```python
from build123d import *

# Parameters (mm, degrees)
CUT_EXTRUDE1_REACH = 60.936
SKETCH2_R          = 2.5


with BuildPart() as part:
    # Sketch1 → Revolve1 (revolve)
    with BuildSketch(Plane(origin=(0, 0, 0), x_dir=(1, 0, 0), z_dir=(0, 1, 0)), mode=Mode.PRIVATE) as revolve1_sk:
        Polygon((0, 0), (0, 28.5), (4, 28.5), (4, 14), (19, 14), (19, 6), (43, 6), (43, 0), align=None)
    revolve(revolve1_sk.sketch.rotate(Axis((-51.704391892, 0, 0), (1, 0, 0)), 180), axis=Axis((-51.704391892, 0, 0), (1, 0, 0)))

    # Sketch2 → Cut-Extrude1 (cut, up to next)
    with BuildSketch(Plane.ZY, mode=Mode.PRIVATE) as cut_extrude1_sk1:
        with Locations((0, 23.75)):
            Circle(SKETCH2_R)
    cut_extrude1_tool1 = extrude(cut_extrude1_sk1.sketch, amount=-CUT_EXTRUDE1_REACH, mode=Mode.PRIVATE) & part.part
    # Sketch2 → Cut-Extrude1 (cut, up to next)
    with BuildSketch(Plane.ZY, mode=Mode.PRIVATE) as cut_extrude1_sk2:
        with Locations((20.56810334, 11.875)):
            Circle(SKETCH2_R)
    cut_extrude1_tool2 = extrude(cut_extrude1_sk2.sketch, amount=-CUT_EXTRUDE1_REACH, mode=Mode.PRIVATE) & part.part
    # Sketch2 → Cut-Extrude1 (cut, up to next)
    with BuildSketch(Plane.ZY, mode=Mode.PRIVATE) as cut_extrude1_sk3:
        with Locations((20.56810334, -11.875)):
            Circle(SKETCH2_R)
    cut_extrude1_tool3 = extrude(cut_extrude1_sk3.sketch, amount=-CUT_EXTRUDE1_REACH, mode=Mode.PRIVATE) & part.part
    # Sketch2 → Cut-Extrude1 (cut, up to next)
    with BuildSketch(Plane.ZY, mode=Mode.PRIVATE) as cut_extrude1_sk4:
        with Locations((0, -23.75)):
            Circle(SKETCH2_R)
    cut_extrude1_tool4 = extrude(cut_extrude1_sk4.sketch, amount=-CUT_EXTRUDE1_REACH, mode=Mode.PRIVATE) & part.part
    # Sketch2 → Cut-Extrude1 (cut, up to next)
    with BuildSketch(Plane.ZY, mode=Mode.PRIVATE) as cut_extrude1_sk5:
        with Locations((-20.56810334, -11.875)):
            Circle(SKETCH2_R)
    cut_extrude1_tool5 = extrude(cut_extrude1_sk5.sketch, amount=-CUT_EXTRUDE1_REACH, mode=Mode.PRIVATE) & part.part
    # Sketch2 → Cut-Extrude1 (cut, up to next)
    with BuildSketch(Plane.ZY, mode=Mode.PRIVATE) as cut_extrude1_sk6:
        with Locations((-20.56810334, 11.875)):
            Circle(SKETCH2_R)
    cut_extrude1_tool6 = extrude(cut_extrude1_sk6.sketch, amount=-CUT_EXTRUDE1_REACH, mode=Mode.PRIVATE) & part.part
    add(cut_extrude1_tool1.solids().sort_by_distance((0, 23.75, 0))[0], mode=Mode.SUBTRACT)
    add(cut_extrude1_tool2.solids().sort_by_distance((0, 11.875, 20.568103))[0], mode=Mode.SUBTRACT)
    add(cut_extrude1_tool3.solids().sort_by_distance((0, -11.875, 20.568103))[0], mode=Mode.SUBTRACT)
    add(cut_extrude1_tool4.solids().sort_by_distance((0, -23.75, 0))[0], mode=Mode.SUBTRACT)
    add(cut_extrude1_tool5.solids().sort_by_distance((0, -11.875, -20.568103))[0], mode=Mode.SUBTRACT)
    add(cut_extrude1_tool6.solids().sort_by_distance((0, 11.875, -20.568103))[0], mode=Mode.SUBTRACT)


solid = part.part
```
Input: part model. Units: mm. Frame: model coordinates. A direction names the side the tool comes from. Give positions to 0.01 mm unless a question says otherwise; leave off trailing zeros. Loops run counter-clockwise (first coordinate to the right, second up) from the corner with the lowest first, then second, coordinate; pieces in that order, holes last.
1) Section query C-C on y = 23.75. Return the cut outline in (x, z).
A:
outline: (0, -15.75) - (4, -15.75) - (4, -2.5) - (0, -2.5) - close; (0, 2.5) - (4, 2.5) - (4, 15.75) - (0, 15.75) - close
2) Line query: L1, parallel to X at y = -15, z = 14.5; L2, parallel to X at y = 2, z = 9; L3, parallel to Z at x = 28, y = 4. Output: solid intervals per line, ascending.
A:
L1: x = 0 to 4
L2: x = 0 to 19
L3: z = -4.47 to 4.47
3) Mould query, pull axis Z, two halves, no side actions, for faces 1 (the flat face through (0, 0, 0)), 2 (the cylindrical face through (1.972, 9.657, 21.722)), 3 (the cylindrical face through (11.605, 5.362, 12.932)). Classes: released by +Z, released by -Z, zero draft, split by the parting line, or undercut.
A:
face 1: zero draft
face 2: undercut
face 3: split by the parting line
4) Section query B-B on y = 0. Return the cut outline in (x, z).
A:
outline: (0, -28.5) - (4, -28.5) - (4, -14) - (19, -14) - (19, -6) - (43, -6) - (43, 6) - (19, 6) - (19, 14) - (4, 14) - (4, 28.5) - (0, 28.5) - close
5) Section query D-D on x = 8. Return the cut outline in (y, z).
A:
outline: circle Ø28 at (0, 0)
6) Section query A-A on z = 0. Return the cut outline in (x, y).
A:
outline: (0, -28.5) - (4, -28.5) - (4, -26.25) - (0, -26.25) - close; (0, -21.25) - (4, -21.25) - (4, -14) - (19, -14) - (19, -6) - (43, -6) - (43, 6) - (19, 6) - (19, 14) - (4, 14) - (4, 21.25) - (0, 21.25) - close; (0, 26.25) - (4, 26.25) - (4, 28.5) - (0, 28.5) - close
7) Contact query for flat-ended pins moving along their axis: pin 1 (3 mm diameter, centred on y = -21, z = -21, fed in from +X); pin 2 (6 mm diameter, centred on x = 15, y = -4.5, fed in from -Z); pin 3 (3 mm diameter, centred on x = 23, y = 3, fed in from -Z). Output: stop coordinate, or through.
A:
pin 1: stops at x = 4
pin 2: stops at z = -13.92
pin 3: stops at z = -5.81
8) Reachability of faces 4 (the flat face through (19, 6, 3)), 5 (the cylindrical face through (1.97, -13.4, -22.55)) from +Z, -Z, +X, -X, +Y, -Y: full face, straight path, thin tool, end or side. Return the list, or none.
A:
face 4: +X
face 5: +X, -X
